Design review of the part built by this model. Coordinates are the model's own, in mm. A direction names the side the tool comes from. Give positions to 0.01 mm unless a question says otherwise; leave off trailing zeros. Write each loop counter-clockwise with the first axis right and the second up, starting at its lowest first coordinate (ties: lowest second). Pieces come first, ordered by that corner, then holes. Notation, with made-up numbers: (-7.75, 84.25) -> (18.25, 84.25) arc R14 ccw to (18.25, 100.25) -> close; hole circle Ø7 at (50, -20). An arc over 180 degrees is marked (long way). Answer as a JSON object with one key per item and string values.
```python
from build123d import *

# Parameters (mm, degrees)
ESQUISSE1_W                = 42
ESQUISSE1_H                = 25.5
BOSS_EXTRU_1_DEPTH         = 6.5
ESQUISSE2_W                = 16
ESQUISSE2_H                = 15
ENL_V_MAT_EXTRU_1_DEPTH    = 10
ESQUISSE3_W                = 5
ESQUISSE3_H                = 25.5
BOSS_EXTRU_2_DEPTH         = 13.5
ESQUISSE6_W                = 5
ESQUISSE6_H                = 29.5
BOSS_EXTRU_3_DEPTH         = 45.5
ESQUISSE4_R                = 1.2
ENL_V_MAT_EXTRU_3_DEPTH    = 45.5
BOSS_EXTRU_4_START         = 22
BOSS_EXTRU_4_DEPTH         = 16
CONG_2_R                   = 5
BOSS_EXTRU_5_DEPTH         = 5
ESQUISSE10_R               = 1.9
ENL_V_MAT_EXTRU_5_DEPTH    = 17
ESQUISSE11_W               = 20
ESQUISSE11_H               = 5
BOSS_EXTRU_6_DEPTH         = 4
BOSS_EXTRU_7_DEPTH         = 5
BOSS_EXTRU_8_DEPTH         = 5.25
R_P_TITION_LIN_AIRE1_COUNT = 2
R_P_TITION_LIN_AIRE1_PITCH = 20.25
ESQUISSE15_W               = 5
ESQUISSE15_H               = 22
BOSS_EXTRU_9_DEPTH         = 10
ESQUISSE16_R               = 1.9
BOSS_EXTRU_10_DEPTH        = 5
R_P_TITION_LIN_AIRE2_COUNT = 2
R_P_TITION_LIN_AIRE2_PITCH = 17


with BuildPart() as part:
    # Esquisse1 → Boss.-Extru.1 (new body)
    with BuildSketch(Plane(origin=(0, 0, 0), x_dir=(1, 0, 0), z_dir=(0, 1, 0))):
        Rectangle(ESQUISSE1_W, ESQUISSE1_H)
    extrude(amount=BOSS_EXTRU_1_DEPTH)

    # Esquisse2 → Enlèv. mat.-Extru.1 (cut)
    with BuildSketch(Plane(origin=(0, 0, 0), x_dir=(1, 0, 0), z_dir=(0, 1, 0))):
        with Locations((-21, 0)):
            Rectangle(ESQUISSE2_W, ESQUISSE2_H)
        with Locations((21, 0)):
            Rectangle(ESQUISSE2_W, ESQUISSE2_H)
    extrude(amount=ENL_V_MAT_EXTRU_1_DEPTH, mode=Mode.SUBTRACT)

    # Esquisse3 → Boss.-Extru.2 (add)
    with BuildSketch(Plane(origin=(0, 6.5, 0), x_dir=(1, 0, 0), z_dir=(0, 1, 0))):
        with Locations((-3.3, 0)):
            Rectangle(ESQUISSE3_W, ESQUISSE3_H)
    extrude(amount=BOSS_EXTRU_2_DEPTH)

    # Esquisse6 → Boss.-Extru.3 (add)
    with BuildSketch(Plane(origin=(0, 20, 0), x_dir=(1, 0, 0), z_dir=(0, 1, 0))):
        with Locations((-3.3, 0)):
            Rectangle(ESQUISSE6_W, ESQUISSE6_H)
    extrude(amount=BOSS_EXTRU_3_DEPTH)

    # Esquisse4 → Enlèv. mat.-Extru.3 (cut)
    with BuildSketch(Plane(origin=(-0.8, 0, 0), x_dir=(0, 0, -1), z_dir=(1, 0, 0))):
        with Locations((-6.3, 52.5)):
            Circle(ESQUISSE4_R)
        with Locations((6.3, 52.5)):
            Circle(ESQUISSE4_R)
        with Locations((6.3, 44.5)):
            Circle(ESQUISSE4_R)
        with Locations((-6.3, 44.5)):
            Circle(ESQUISSE4_R)
    extrude(amount=-ENL_V_MAT_EXTRU_3_DEPTH, mode=Mode.SUBTRACT)

    # Esquisse5 → Boss.-Extru.4 (add)
    with BuildSketch(Plane(origin=(0, 20, 0), x_dir=(1, 0, 0), z_dir=(0, 1, 0)).offset(BOSS_EXTRU_4_START)):
        Polygon((-0.8, 14.75), (-0.8, 12), (12.7, 12), (12.7, -12), (-0.8, -12), (-0.8, -14.75), (15.7, -14.75), (15.7, 14.75), align=None)
    extrude(amount=BOSS_EXTRU_4_DEPTH)

    # Congé2
    cong_2_edges = [part.edges().sort_by_distance(p)[0] for p in [
        (-0.8, 42, 13.375),
        (-0.8, 42, -13.375),
    ]]
    fillet(cong_2_edges, radius=CONG_2_R)

    # Esquisse9 → Boss.-Extru.5 (add)
    with BuildSketch(Plane.XY.offset(12.75)):
        Polygon((-0.8, 22.034425492), (-0.8, 6.5), (11.926120582, 6.5), (-0.8, 31.53809605), align=None)
    extrude(amount=-BOSS_EXTRU_5_DEPTH)

    # Esquisse10 → Enlèv. mat.-Extru.5 (cut)
    with BuildSketch(Plane(origin=(0, 6.5, 0), x_dir=(1, 0, 0), z_dir=(0, 1, 0))):
        with Locations(Location((-9.199739461, 0, 0), (0, 0, 270))):
            Circle(ESQUISSE10_R)
        with Locations(Location((4.800260539, 0, 0), (0, 0, 270))):
            Circle(ESQUISSE10_R)
    extrude(amount=-ENL_V_MAT_EXTRU_5_DEPTH, mode=Mode.SUBTRACT)

    # Esquisse11 → Boss.-Extru.6 (add)
    with BuildSketch(Plane.ZY.offset(5.8)):
        with Locations((0, 37.55)):
            Rectangle(ESQUISSE11_W, ESQUISSE11_H)
    extrude(amount=BOSS_EXTRU_6_DEPTH)

    # Esquisse12 → Boss.-Extru.7 (add)
    with BuildSketch(Plane(origin=(0, 0, -12.75), x_dir=(-1, 0, 0), z_dir=(0, 0, -1))):
        Polygon((0.8, 21.304240475), (-11.926120582, 6.5), (0.8, 6.5), align=None)
    extrude(amount=-BOSS_EXTRU_7_DEPTH)

    # Esquisse13 → Boss.-Extru.8 (add)
    with BuildSketch(Plane.XY.offset(12.75)):
        Polygon((-21, 6.5), (-5.8, 31.179013399), (-5.8, 6.5), align=None)
    boss_extru_8 = extrude(amount=-BOSS_EXTRU_8_DEPTH)

    # Répétition linéaire1: Boss.-Extru.8 ×2
    with Locations(*[(0, 0, -i * R_P_TITION_LIN_AIRE1_PITCH) for i in range(1, R_P_TITION_LIN_AIRE1_COUNT)]):
        add(boss_extru_8)

    # Esquisse15 → Boss.-Extru.9 (add)
    with BuildSketch(Plane(origin=(0, 65.5, 0), x_dir=(1, 0, 0), z_dir=(0, 1, 0))):
        with Locations((-3.3, 0)):
            Rectangle(ESQUISSE15_W, ESQUISSE15_H)
    extrude(amount=BOSS_EXTRU_9_DEPTH)

    # Esquisse16 → Boss.-Extru.10 (add)
    with BuildSketch(Plane.XY.offset(11)):
        with BuildLine():
            Line((-5.8, 75.5), (-5.8, 67.5))
            Line((-5.8, 67.5), (-13.8, 67.5))
            ThreePointArc((-13.8, 67.5), (-15.214213562, 68.085786438), (-15.8, 69.5))
            Line((-15.8, 69.5), (-15.8, 73.5))
            ThreePointArc((-15.8, 73.5), (-15.214213562, 74.914213562), (-13.8, 75.5))
            Line((-13.8, 75.5), (-5.8, 75.5))
        make_face()
        with Locations((-12.3, 71.5)):
            Circle(ESQUISSE16_R, mode=Mode.SUBTRACT)
    boss_extru_10 = extrude(amount=-BOSS_EXTRU_10_DEPTH)

    # Répétition linéaire2: Boss.-Extru.10 ×2
    with Locations(*[(0, 0, -i * R_P_TITION_LIN_AIRE2_PITCH) for i in range(1, R_P_TITION_LIN_AIRE2_COUNT)]):
        add(boss_extru_10)


solid = part.part
```
(1) The part is to be moulded in two halves that separate along Z. For faces 1 (the flat face through (21, 3, 10)), 2 (the flat face through (-7, 72, 11)), 3 (the flat face through (-10, 72, -6)), say which applies: +Z half, -Z half, draft (parallel to the pull), parting line (faces both ways), or undercut.
Here are the results:
{"face 1": "draft", "face 2": "+Z half", "face 3": "undercut"}
(2) We need section C-C, the plane y = 44.5. State the section outline as (x, z) points.
Here are the results:
{"outline": "(-5.8, -14.75) -> (15.7, -14.75) -> (15.7, 14.75) -> (-5.8, 14.75) -> (-5.8, 7.5) -> (-0.8, 7.5) -> (-0.8, 12) -> (12.7, 12) -> (12.7, -12) -> (-0.8, -12) -> (-0.8, -7.5) -> (-5.8, -7.5) -> close; (-5.8, -5.1) -> (-0.8, -5.1) -> (-0.8, 5.1) -> (-5.8, 5.1) -> close"}
(3) We need section A-A, the plane z = -3. State the section outline as (x, y) points, then the cut area to 3 significant figures.
Here are the results:
{"outline": "(-13, 0) -> (13, 0) -> (13, 6.5) -> (-0.8, 6.5) -> (-0.8, 75.5) -> (-5.8, 75.5) -> (-5.8, 40.05) -> (-9.8, 40.05) -> (-9.8, 35.05) -> (-5.8, 35.05) -> (-5.8, 6.5) -> (-13, 6.5) -> close; (12.7, 42) -> (15.7, 42) -> (15.7, 58) -> (12.7, 58) -> close", "area": "582 mm²"}
(4) Clearance check with flat-ended pins moving along their axes: pin 1 (3 mm diameter, centred on x = -9.2, z = 0, fed in from -Y); pin 2 (2 mm diameter, centred on x = -8.5, y = 36.5, fed in from -Z); pin 3 (4 mm diameter, centred on y = 52.5, z = -6.3, fed in from +X). State where each tip first meets the part, or that it passes through.
Here are the results:
{"pin 1": "stops at y = 35.05", "pin 2": "stops at z = -10", "pin 3": "stops at x = 15.7"}
(5) We need section B-B, the plane y = 71.5. State the section outline as (x, z) points.
Here are the results:
{"outline": "(-15.8, -11) -> (-14.2, -11) -> (-14.2, -6) -> (-15.8, -6) -> close; (-15.8, 6) -> (-14.2, 6) -> (-14.2, 11) -> (-15.8, 11) -> close; (-10.4, -11) -> (-0.8, -11) -> (-0.8, 11) -> (-10.4, 11) -> (-10.4, 6) -> (-5.8, 6) -> (-5.8, -6) -> (-10.4, -6) -> close"}
(6) We need section D-D, the plane z = 0.75. State the section outline as (x, y) points, then the cut area to 3 significant figures.
Here are the results:
{"outline": "(-13, 0) -> (-10.95, 0) -> (-10.95, 6.5) -> (-13, 6.5) -> close; (-9.8, 35.05) -> (-5.8, 35.05) -> (-5.8, 6.5) -> (-7.45, 6.5) -> (-7.45, 0) -> (3.05, 0) -> (3.05, 6.5) -> (-0.8, 6.5) -> (-0.8, 75.5) -> (-5.8, 75.5) -> (-5.8, 40.05) -> (-9.8, 40.05) -> close; (6.55, 0) -> (13, 0) -> (13, 6.5) -> (6.55, 6.5) -> close; (12.7, 42) -> (15.7, 42) -> (15.7, 58) -> (12.7, 58) -> close", "area": "537 mm²"}
(7) For faces 4 (the flat face through (17, 3, -7.5)), 5 (the flat face through (6, 50, 12)), 6 (the flat face through (3, 14, 7.75)), 7 (the flat face through (-3, 20, -14)), 8 (the flat face through (-8, 38, 10)), list the 3-axis set-ups (+Z, -Z, +X, -X, +Y, -Y) from which the entire face can be reached by the end or side of a thin tool; tool diameter is ignored.
Here are the results:
{"face 4": "+X, -Y", "face 5": "+Y", "face 6": "+X, +Y", "face 7": "-Z, +X, -X, -Y", "face 8": "+Z, -X"}
(8) For line 1 along X through (y, z) = (3.5, 0); line 2 along Y through (x, z) = (-3.95, 6.3); line 3 along X through (y, z) = (47, 1.75), list the stretches that pass through material, from the lowest coordinate up.
Here are the results:
{"line 1": "x = -13 to -11.1, -7.3 to 2.9, 6.7 to 13", "line 2": "y = 0 to 43.3, 45.7 to 51.3, 53.7 to 75.5", "line 3": "x = -5.8 to -0.8, 12.7 to 15.7"}
